Geometry: see drawing. Coordinates: mm, zero at the bounding-box minimum. A direction names the side the tool comes from. Round coordinates to 2 decimals unless told otherwise and drop trailing zeros. Order: outer loops, then holes, each group sorted by start corner. A loop starts at its lowest first (then second) coordinate and runs counter-clockwise, first axis right, second up. Notation, with made-up numbers: (-14, -32.5) -> (7, -32.5) arc R25 ccw to (7, -1.5) -> close; hole circle Ø3 at (38.5, 53). An arc over 180 degrees is marked (long way). Answer as CSV lines item,"result". Start each with the question number.
(1) Section query C-C (x = 21.5). Count the separate pieces of the cut face and the enclosed holes in it.
(2) Line query: line 1 along X through (y, z) = (4.45, 10); line 2 along Y through (x, z) = (13.5, 2.4); line 3 along Y through (x, z) = (21.5, 1.9). Output: solid intervals per line, ascending. Write a range as from..to.
(3) Contact query for flat-ended pins moving along their axis: P1, Ø1.8, axis at x = 31, z = 8.5, coming from the +Y side; P2, Ø10, axis at x = 10.5, z = 15, coming from the +Y side; P3, Ø8, axis at x = 19.5, y = 18.5, coming from the +Z side. Output: stop coordinate, or through.
(4) Section query B-B (y = 26.5). Output: boundary loops of the cut face in (x, z).
(5) Section query D-D (z = 10.75). Output: boundary loops of the cut face in (x, y) (1 decimal).
(6) Pull-direction query (X, two-part tool) for the marked faces 1, 2 and 3; classes: +X half, -X half, draft (parallel to the pull), parting line (faces both ways), or undercut.
(7) Set-up query: the marked faces 4, 5 and 6. Return all of +Z, -Z, +X, -X, +Y, -Y with unobstructed straight access to the full face (end or side cutting, diameter ignored); none if empty.
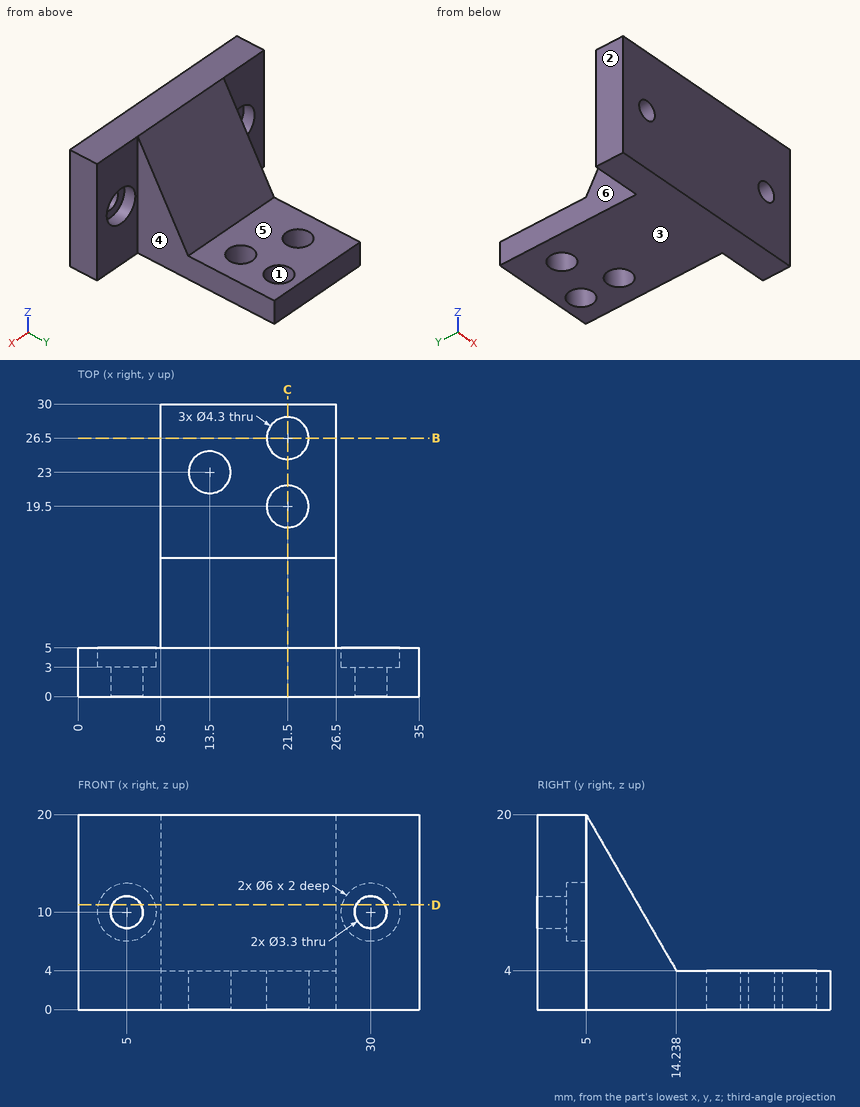
Answer block:
1,separate pieces,"3"
1,enclosed holes,"0"
2,line 1,"0..2, 8..27, 33..35"
2,line 2,"0..20.85, 25.15..30"
2,line 3,"0..17.35, 21.65..24.35, 28.65..30"
3,P1,"y = 3"
3,P2,"y = 10.77"
3,P3,"z = 4"
4,outline,"(8.5, 0) -> (19.35, 0) -> (19.35, 4) -> (8.5, 4) -> close; (23.65, 0) -> (26.5, 0) -> (26.5, 4) -> (23.65, 4) -> close"
5,outline,"(0, 0) -> (3.5, 0) -> (3.5, 3) -> (2.1, 3) -> (2.1, 5) -> (0, 5) -> close; (6.5, 0) -> (28.5, 0) -> (28.5, 3) -> (27.1, 3) -> (27.1, 5) -> (26.5, 5) -> (26.5, 10.3) -> (8.5, 10.3) -> (8.5, 5) -> (7.9, 5) -> (7.9, 3) -> (6.5, 3) -> close; (31.5, 0) -> (35, 0) -> (35, 5) -> (32.9, 5) -> (32.9, 3) -> (31.5, 3) -> close"
6,face 1,"undercut"
6,face 2,"-X half"
6,face 3,"draft"
7,face 4,"+Z, -Z, +X, +Y"
7,face 5,"+Z, +X, -X, +Y"
7,face 6,"+Z, -Z, -X, +Y"
